CAD build for the part. Positions are in the model's coordinates, mm. A direction names the side the tool comes from. Round coordinates to 2 decimals unless told otherwise and drop trailing zeros. Write each loop counter-clockwise with the first axis right and the second up, starting at its lowest first coordinate (ties: lowest second). Pieces come first, ordered by that corner, then holes. Notation, with made-up numbers: (41.25, 52.5) -> (45.25, 52.5) arc R27 ccw to (45.25, 71.5) -> close; hole circle Ø3 at (26, 12.5). An arc over 180 degrees is marked (long way). Answer in a Markdown table with one row per item. Add a question column.
```python
from build123d import *

# Parameters (mm, degrees)
SKETCH1_W           = 48.5
SKETCH1_H           = 45
BOSS_EXTRUDE1_DEPTH = 3
CUT_EXTRUDE1_DEPTH  = 4
FILLET1_R           = 5


with BuildPart() as part:
    # Sketch1 → Boss-Extrude1 (new body)
    with BuildSketch(Plane(origin=(0, 0, 0), x_dir=(0, 0, -1), z_dir=(1, 0, 0))):
        with Locations((24.25, 22.5)):
            Rectangle(SKETCH1_W, SKETCH1_H)
    extrude(amount=BOSS_EXTRUDE1_DEPTH)

    # Sketch2 → Cut-Extrude1 (cut, through all)
    with BuildSketch(Plane(origin=(3, 0, 0), x_dir=(0, 0, -1), z_dir=(1, 0, 0))):
        with BuildLine():
            Line((25.3, 35), (25.3, 0))
            Line((25.3, 0), (31.1, 0))
            Line((31.1, 0), (31.1, 35))
            ThreePointArc((31.1, 35), (28.2, 37.9), (25.3, 35))
        make_face()
    extrude(amount=-CUT_EXTRUDE1_DEPTH, mode=Mode.SUBTRACT)

    # Fillet1
    fillet1_edges = [part.edges().sort_by_distance(p)[0] for p in [
        (1.5, 45, 0),
        (1.5, 45, -48.5),
    ]]
    fillet(fillet1_edges, radius=FILLET1_R)


solid = part.part
```
Item 1: Drill centre lines: probe 1 along Z at (x, y) = (0.6, 9); probe 2 along Y at (x, z) = (2.05, -30); probe 3 along Y at (x, z) = (2.3, -44). Where is each one in solid material? Low to high.
Item 2: Tool access for faces 1 (the flat face through (1, 0, -40)), 2 (the flat face through (2, 18, -25.3)): list every direction of +Z, -Z, +X, -X, +Y, -Y with a clear straight run to the whole face (end or side of a thin tool).
Item 3: Two-plate mould, pull along Z, no slides. Class faces 3 (the flat face through (3, 23, -24)), 4 (the flat face through (2, 17, -31.1)), 5 (the cylindrical face through (1.5, 37.9, -28.3)), 6 (the cylindrical face through (2, 43, -1)): +Z half, -Z half, draft (parallel to the pull), parting line (faces both ways), or undercut.
Item 4: Saw through at B-B on x = 2.55. Give the cut face in (y, z), then the cut area to 3 significant figures.
Item 5: Saw through at A-A on y = 17. Give the cut face in (x, z).
Item 6: Pin check, flat tip, straight feed: pin 1 (6 mm diameter, centred on y = 32, z = -10.5, fed in from -X). Stop position of the tip, or through.
Item 7: Saw through at C-C on z = -28.2. Give the cut face in (x, y).
Recorded:
| question | item | result |
|---|---|---|
| 1 | probe 1 | -48.5 to -31.1, -25.3 to 0 |
| 1 | probe 2 | 37.27 to 45 |
| 1 | probe 3 | 0 to 44.97 |
| 2 | face 1 | +Z, -Z, +X, -X, -Y |
| 2 | face 2 | +X, -X, -Y |
| 3 | face 3 | draft |
| 3 | face 4 | undercut |
| 3 | face 5 | undercut |
| 3 | face 6 | +Z half |
| 4 | outline | (0, -48.5) -> (40, -48.5) arc R5 ccw to (45, -43.5) -> (45, -5) arc R5 ccw to (40, 0) -> (0, 0) -> (0, -25.3) -> (35, -25.3) arc R2.9 cw to (35, -31.1) -> (0, -31.1) -> close |
| 4 | area | 1,960 mm2 |
| 5 | outline | (0, -48.5) -> (3, -48.5) -> (3, -31.1) -> (0, -31.1) -> close; (0, -25.3) -> (3, -25.3) -> (3, 0) -> (0, 0) -> close |
| 6 | pin 1 | x = 0 |
| 7 | outline | (0, 37.9) -> (3, 37.9) -> (3, 45) -> (0, 45) -> close |
